Source: CAD feature listing. Evaluate the final solid. Frame: model axes, mm. Face numbers are marked on the shaded views. Coordinates: 2 decimals unless noted, no trailing zeros. Write each loop counter-clockwise with the first axis right and the second up, starting at its lowest first coordinate (ties: lowest second). Pieces come first, ordered by that corner, then holes. Notation, with made-up numbers: (-5, 31.25) - (15, 31.25) arc R25 cw to (15, 50.25) - close; hole circle Ø5 at (15, 10). An arc over 180 degrees is marked (long way). One line per item, written item: value.
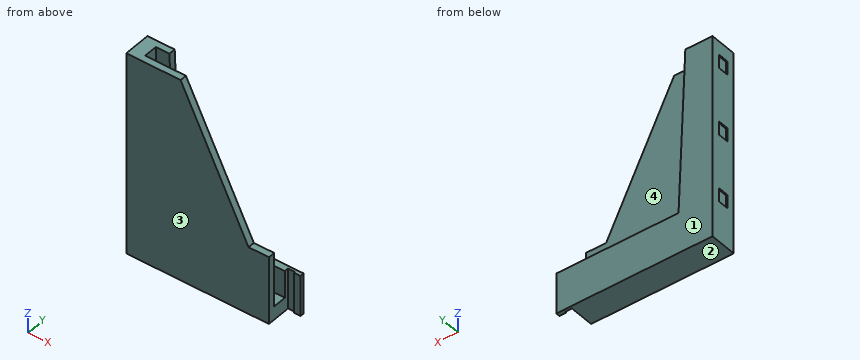
from build123d import *

# Parameters (mm, degrees)
F0_W      = 95
F0_H      = 5
F1_DEPTH  = 50
F2_W      = 95
F2_H      = 10
F3_DEPTH  = 10
F4_W      = 5
F4_H      = 2
F5_DEPTH  = 30
F6_W      = 10
F6_H      = 120
F7_DEPTH  = 5
F8_W      = 30
F8_H      = 100
F9_DEPTH  = 5
F10_W     = 10
F10_H     = 20
F11_DEPTH = 150
F12_W     = 8
F12_H     = 10
F13_DEPTH = 1


with BuildPart() as f1:
    # F0 (on Top) → F1 (new body)
    with BuildSketch(Plane.XY):
        with Locations((47.5, 2.5)):
            Rectangle(F0_W, F0_H)
    extrude(amount=F1_DEPTH)

    # F2 (on Top) → F3 (join)
    with BuildSketch(Plane.XY):
        with Locations((47.5, 10)):
            Rectangle(F2_W, F2_H)
    extrude(amount=F3_DEPTH)

    # F4 (on Top) → F5 (join)
    with BuildSketch(Plane.XY):
        Polygon((0, 20), (0, 15), (95, 15), (95, 18), (95, 20), align=None)
        with Locations((97.5, 19)):
            Rectangle(F4_W, F4_H)
        Polygon((100, 20), (100, 18), (100, 17), (105, 17), (105, 20), align=None)
    extrude(amount=F5_DEPTH)

    # F6 (on face) → F7 (join)
    with BuildSketch(Plane(origin=(0, 20, 0), x_dir=(-1, 0, 0), z_dir=(0, 1, 0))):
        with Locations((-5, 90)):
            Rectangle(F6_W, F6_H)
        Polygon((-15, 30), (-10, 30), (-10, 150), align=None)
    extrude(amount=-F7_DEPTH)

    # F8 (on face) → F9 (join)
    with BuildSketch(Plane.XZ):
        with Locations((15, 100)):
            Rectangle(F8_W, F8_H)
        Polygon((30, 150), (30, 50), (80, 50), align=None)
    extrude(amount=-F9_DEPTH)

    # F10 (on Top) → F11 (join)
    with BuildSketch(Plane.XY):
        with Locations((-5, 10)):
            Rectangle(F10_W, F10_H)
    extrude(amount=F11_DEPTH)

    # F12 (on face) → F13 (cut)
    with BuildSketch(Plane(origin=(-10, 0, 0), x_dir=(0, -1, 0), z_dir=(-1, 0, 0))):
        with Locations((-10, 135)):
            Rectangle(F12_W, F12_H)
        with Locations((-10, 85)):
            Rectangle(F12_W, F12_H)
        with Locations((-10, 35)):
            Rectangle(F12_W, F12_H)
    extrude(amount=-F13_DEPTH, mode=Mode.SUBTRACT)


solid = f1.part
1) Section query C-C on z = 18. Output: boundary loops of the cut face in (x, y).
Values found:
outline: (-10, 0) - (95, 0) - (95, 5) - (0, 5) - (0, 15) - (95, 15) - (95, 18) - (100, 18) - (100, 17) - (105, 17) - (105, 20) - (-10, 20) - close
2) Material intervals for line 1 (Y direction, x = 8, z = 131); line 2 (Y direction, x = 78.5, z = 42); line 3 (X direction, y = 9.75, z = 143), sorted ascending.
Values found:
line 1: 0 to 5, 15 to 20
line 2: 0 to 5
line 3: -10 to 0
3) Section query D-D on x = 21. Output: boundary loops of the cut face in (y, z).
Values found:
outline: (0, 0) - (20, 0) - (20, 30) - (15, 30) - (15, 10) - (5, 10) - (5, 150) - (0, 150) - close
4) Section query B-B on y = 8.5. Output: boundary loops of the cut face in (x, z), then the cut area to 3 significant figures.
Values found:
outline: (-10, 0) - (95, 0) - (95, 10) - (0, 10) - (0, 150) - (-10, 150) - (-10, 140) - (-9, 140) - (-9, 130) - (-10, 130) - (-10, 90) - (-9, 90) - (-9, 80) - (-10, 80) - (-10, 40) - (-9, 40) - (-9, 30) - (-10, 30) - close
area: 2,420 mm2
5) Section query A-A on x = 61.5. Output: boundary loops of the cut face in (y, z).
Values found:
outline: (0, 0) - (20, 0) - (20, 30) - (15, 30) - (15, 10) - (5, 10) - (5, 87) - (0, 87) - close
6) Draft query along Y for the marked faces 1, 2, 3 and 4. Return one class per face: released by +Y, released by -Y, zero draft, split by the parting line, or undercut.
Values found:
face 1: released by +Y
face 2: zero draft
face 3: released by -Y
face 4: undercut
7) Contact query for flat-ended pins moving along their axis: P1, Ø3, axis at y = 12.5, z = 90.5, coming from the +X side; P2, Ø5, axis at y = 2, z = 71.5, coming from the +X side; P3, Ø5, axis at x = 15.5, z = 86, coming from the +Y side. Output: stop coordinate, or through.
Values found:
P1: x = 0
P2: x = 70.5
P3: y = 5
